Autodesk Inventor part; units mm, degrees
ref_plane "YZ Plane" through (0, 0, 0) normal (1, 0, 0) x (0, 1, 0)
ref_plane "XZ Plane" through (0, 0, 0) normal (0, 1, 0) x (-1, 0, 0)
ref_plane "XY Plane" through (0, 0, 0) normal (0, 0, 1) x (1, 0, 0)
sketch "스케치1" plane through (0, 0, 0) normal (0, 0, 1) x (1, 0, 0)
  line L0 (0, 0) -> (2.5, 0)
  line L1 (0, 0) -> (0, 8.7)
  line L2 (2.5, 0) -> (2.7, 0)
  line L3 (2.7, 0) -> (2.7, 1)
  line L4 (2.7, 1) -> (2.5, 1)
  line L5 (2.5, 1) -> (2.5, 6.2)
  line L6 (2.5, 8.7) -> (0, 8.7)
  arc A0 (2.5, 6.2) -> (0, 8.7) centre (0, 6.2) ccw
  dimension "d0" = 2.5
  dimension "d1" = 8.7
  dimension "d2" = 0.2
  dimension "d3" = 1
  dimension "d4" = 2.5
revolve "회전1" add sketch "스케치1" angle 360 about axis through (0, 0, 0) along (0, 1, 0)
sketch "스케치2" plane through (0, 0, 0) normal (1, 0, 0) x (0, 1, 0)
  line L0 (0, 2.7) -> (0, -2.7)
  line L1 (0, -1.56) -> (-6.3813, -1.56)
  line L2 (-6.3813, -1.56) -> (-6.3813, -1.06)
  line L3 (-6.3813, -1.06) -> (0, -1.06)
  line L4 (0, -1.06) -> (0, -1.56)
  line L5 (0, 1.56) -> (-10.1722, 1.56)
  line L6 (-10.1722, 1.56) -> (-10.1722, 1.06)
  line L7 (-10.1722, 1.06) -> (0, 1.06)
  line L8 (0, 1.06) -> (0, 1.56)
  point P0 (0, 0)
  point P1 (0, 1.06)
  dimension "d7" = 1.14
  dimension "d8" = 1.14
  dimension "d9" = 0.5
  dimension "d10" = 0.5
extrude "돌출1" add sketch "스케치2" along normal mid plane 0.5
properties part number "LED"
Source: CAD feature listing. Evaluate the final solid. Frame: model axes, mm. A direction names the side the tool comes from. Give positions to 0.01 mm unless a question says otherwise; leave off trailing zeros. Loops run counter-clockwise (first coordinate to the right, second up) from the corner with the lowest first, then second, coordinate; pieces in that order, holes last. Notation, with made-up numbers: (13, -4.75) -> (19, -4.75) arc R24 cw to (19, 14.25) -> close; hole circle Ø6 at (-3.75, -15.75). An arc over 180 degrees is marked (long way). Use a Markdown table: item, result. Add a question column.
(1) Section query D-D (y = 4.25). Output: boundary loops of the cut face in (x, z), then the cut area to 3 significant figures.
(2) Section query C-C (x = 0). Output: boundary loops of the cut face in (y, z), then the cut area to 3 significant figures.
(3) Section query B-B (z = 0). Output: boundary loops of the cut face in (x, y).
(4) First-contact query: pin 1 Ø0.6 at (x, y) = (0, -3) entering from -Z; pin 2 Ø2.5 at (x, z) = (1, -0.5) entering from -Y; pin 3 Ø0.6 at (y, z) = (-3.5, 1.5) entering from +X; pin 4 Ø1.5 at (x, y) = (1.5, -5.5) entering from -Z. Flat tips, straight axial feed; report the tip coordinate or a pass-through.
(5) Section query A-A (y = -4.5). Output: boundary loops of the cut face in (x, z).
(6) Ray query, line 1 (X direction, y = -7.5, z = 1.35); line 2 (Y direction, x = 1.9, z = 1.2); line 3 (Y direction, x = 0.3, z = -2.15). Return the intervals inside material, ascending.
(7) Access query for faces 1 (the face through (-0.585, 0.507, 2.636)), 2 (the face through (-0.54, 3.64, 2.44)). Directions: +Z, -Z, +X, -X, +Y, -Y. A direction counts if a zero-diameter tool reaches every point of the face in a straight line with its end or side. Return the directions, or none.
Checked values:
| question | item | result |
|---|---|---|
| 1 | outline | circle Ø5 at (0, 0) |
| 1 | area | 19.6 mm^2 |
| 2 | outline | (-10.17, 1.06) -> (0, 1.06) -> (0, -1.06) -> (-6.38, -1.06) -> (-6.38, -1.56) -> (0, -1.56) -> (0, -2.7) -> (1, -2.7) -> (1, -2.5) -> (6.2, -2.5) arc R2.5 ccw to (6.2, 2.5) -> (1, 2.5) -> (1, 2.7) -> (0, 2.7) -> (0, 1.56) -> (-10.17, 1.56) -> close |
| 2 | area | 49.5 mm^2 |
| 3 | outline | (-2.7, 0) -> (2.7, 0) -> (2.7, 1) -> (2.5, 1) -> (2.5, 6.2) arc R2.5 ccw to (-2.5, 6.2) -> (-2.5, 1) -> (-2.7, 1) -> close |
| 4 | pin 1 | z = -1.56 |
| 4 | pin 2 | y = -6.38 |
| 4 | pin 3 | x = 0.25 |
| 4 | pin 4 | through |
| 5 | outline | (-0.25, -1.56) -> (0.25, -1.56) -> (0.25, -1.06) -> (-0.25, -1.06) -> close; (-0.25, 1.06) -> (0.25, 1.06) -> (0.25, 1.56) -> (-0.25, 1.56) -> close |
| 6 | line 1 | -0.25 to 0.25 |
| 6 | line 2 | 0 to 7.3 |
| 6 | line 3 | 0 to 7.44 |
| 7 | face 1 | +Y, -Y |
| 7 | face 2 | +Y |
